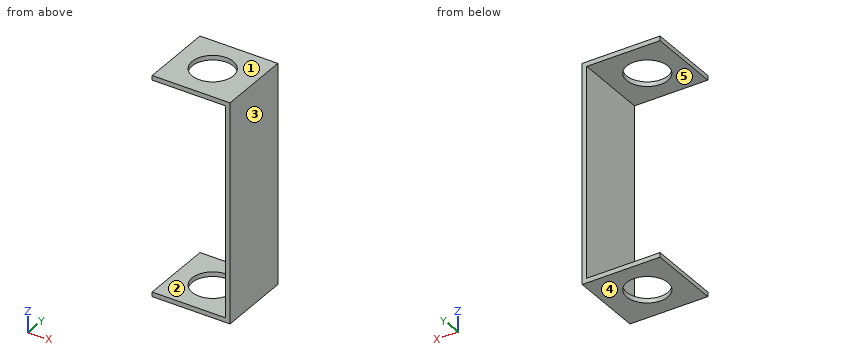
```python
from build123d import *

# Parameters (mm, degrees)
SKETCH1_W           = 53.975
SKETCH1_H           = 50.8
SKETCH1_R           = 14.2875
BOSS_EXTRUDE1_DEPTH = 3.175
SKETCH2_W           = 3.175
SKETCH2_H           = 50.8
BOSS_EXTRUDE2_DEPTH = 146.05
SKETCH3_W           = 3.175
SKETCH3_H           = 50.8
SKETCH3_W_2         = 50.8
SKETCH3_R           = 14.2875
BOSS_EXTRUDE3_DEPTH = 3.175


with BuildPart() as part:
    # Sketch1 → Boss-Extrude1 (new body)
    with BuildSketch(Plane.XY):
        with Locations((26.9875, -25.4)):
            Rectangle(SKETCH1_W, SKETCH1_H)
        with Locations((25.4, -25.4)):
            Circle(SKETCH1_R, mode=Mode.SUBTRACT)
    extrude(amount=BOSS_EXTRUDE1_DEPTH)

    # Sketch2 → Boss-Extrude2 (add)
    with BuildSketch(Plane.XY.offset(3.175)):
        with Locations((52.3875, -25.4)):
            Rectangle(SKETCH2_W, SKETCH2_H)
    extrude(amount=BOSS_EXTRUDE2_DEPTH)

    # Sketch3 → Boss-Extrude3 (add)
    # profile 1 of 2: a face of its own
    with BuildSketch(Plane.XY.offset(149.225)):
        with Locations((52.3875, -25.4)):
            Rectangle(SKETCH3_W, SKETCH3_H)
    # profile 2 of 2: a face of its own
    with BuildSketch(Plane.XY.offset(149.225)):
        with Locations((25.4, -25.4)):
            Rectangle(SKETCH3_W_2, SKETCH3_H)
        with Locations((25.4, -25.4)):
            Circle(SKETCH3_R, mode=Mode.SUBTRACT)
    extrude(amount=BOSS_EXTRUDE3_DEPTH)


solid = part.part
```
Geometry check sheet. Reference: the model listing, model coordinates, mm. Face numbers are marked on the shaded views. A direction names the side the tool comes from. Round coordinates to 2 decimals unless told otherwise and drop trailing zeros. Loops run counter-clockwise (first coordinate to the right, second up) from the corner with the lowest first, then second, coordinate; pieces in that order, holes last. Notation, with made-up numbers: (-10.75, 84) - (47.25, 84) arc R20 cw to (47.25, 121) - close; hole circle Ø2 at (79.25, 18.25). An arc over 180 degrees is marked (long way). Write item = value, one per line. Start each with the question number.
1. Set-up check for the marked faces 4 and 5: record each of +Z, -Z, +X, -X, +Y, -Y from which the full face is reachable in a straight line by a thin tool's end or side.
2. Mould release check, pull along Z, two halves, no side actions. Record for the marked faces 1, 2 and 3: released by +Z, released by -Z, zero draft, split by the parting line, or undercut.
3. Section check C-C on y = -42. Enter the section's corners in (x, z) (3 decimals), then the cut area to 3 significant figures.
4. Thickness scan on line 1 (Y direction, x = 25.4, z = 2.15); line 2 (Z direction, x = 46, y = -37) (3 decimals); line 3 (X direction, y = -25, z = 150) (3 decimals). Record the ranges inside material, lowest first.
5. Section check B-B on x = 25.4. Enter the section's corners in (y, z) (1 decimal), then the cut area to 3 significant figures.
6. Section check A-A on y = -25.4. Enter the section's corners in (x, z) (1 decimal), then the cut area to 3 significant figures.
7. Section check D-D on z = 139. Enter the section's corners in (x, y) (3 decimals).
8. Depth check by flat-ended pin: pin 1 (1.5 mm diameter, centred on y = -23.5, z = 67, fed in from -X); pin 2 (6 mm diameter, centred on x = 35, y = -17, fed in from +Z). Enter the tip coordinate at first touch or a pass-through.
Working result:
q1.face_4 = -Z, +X, -X, +Y, -Y
q1.face_5 = -X, +Y, -Y
q2.face_1 = released by +Z
q2.face_2 = undercut
q2.face_3 = zero draft
q3.outline = (0, 0) - (53.975, 0) - (53.975, 152.4) - (0, 152.4) - (0, 149.225) - (50.8, 149.225) - (50.8, 3.175) - (0, 3.175) - close
q3.area = 806 mm^2
q4.line_1 = -50.8 to -39.69, -11.11 to 0
q4.line_2 = 0 to 3.175, 149.225 to 152.4
q4.line_3 = 0 to 11.118, 39.682 to 53.975
q5.outline = (-50.8, 0) - (-39.7, 0) - (-39.7, 3.2) - (-50.8, 3.2) - close; (-50.8, 149.2) - (-39.7, 149.2) - (-39.7, 152.4) - (-50.8, 152.4) - close; (-11.1, 0) - (0, 0) - (0, 3.2) - (-11.1, 3.2) - close; (-11.1, 149.2) - (0, 149.2) - (0, 152.4) - (-11.1, 152.4) - close
q5.area = 141 mm^2
q6.outline = (0, 0) - (11.1, 0) - (11.1, 3.2) - (0, 3.2) - close; (0, 149.2) - (11.1, 149.2) - (11.1, 152.4) - (0, 152.4) - close; (39.7, 0) - (54, 0) - (54, 152.4) - (39.7, 152.4) - (39.7, 149.2) - (50.8, 149.2) - (50.8, 3.2) - (39.7, 3.2) - close
q6.area = 625 mm^2
q7.outline = (50.8, -50.8) - (53.975, -50.8) - (53.975, 0) - (50.8, 0) - close
q8.pin_1 = 50.8
q8.pin_2 = 152.4
